```python
from build123d import *

# Parameters (mm, degrees)
F0_R     = 12.7
F1_DEPTH = 19.05
F2_R     = 2.54
F3_DEPTH = 12.7
F4_R     = 2.54
F4_R_2   = 2.674386
F5_DEPTH = 12.7


with BuildPart() as f1:
    # F0 (on Right) → F1 (new body)
    with BuildSketch(Plane.YZ):
        Circle(F0_R)
    extrude(amount=F1_DEPTH)

    # F2 (on face) → F3 (join)
    with BuildSketch(Plane.YZ.offset(19.05)):
        Circle(F2_R)
    extrude(amount=F3_DEPTH)

    # F4 (on face) → F5 (join)
    with BuildSketch(Plane(origin=(0, 0, 0), x_dir=(0, -1, 0), z_dir=(-1, 0, 0))):
        with Locations((-5.08, 0)):
            Circle(F4_R)
        with Locations((5.08, 0)):
            Circle(F4_R_2)
    extrude(amount=F5_DEPTH)


solid = f1.part
```
Verification items for the finished model (mm, model axes). A direction names the side the tool comes from. Give positions to 0.01 mm unless a question says otherwise; leave off trailing zeros. Order: outer loops, then holes, each group sorted by start corner. A loop starts at its lowest first (then second) coordinate and runs counter-clockwise, first axis right, second up. Notation, with made-up numbers: M 46,-38.75 L 89,-38.75 A22 ccw 89,-30.75 Z; hole C -33,71 d3. An arc over 180 degrees is marked long. Return JSON: item names as keys, results as strings. Group by question number.
1) Section check B-B on x = 15. Record the cut outline in (y, z).
2) Mould release check, pull along Y, two halves, no side actions. Record for faces 1 (the face through (9.39, -2.75, -12.4)), 2 (the face through (-12.7, 5, 0)), 3 (the face through (-6.261, 7.096, -1.546)): pulls with the +Y half, pulls with the -Y half, needs draft (parallel to the pull), parting line crosses it, or undercut.
3) Section check D-D on y = -5.08. Record the cut outline in (x, z), and give its area (3 significant figures).
4) Go/stop test with flat-tipped pins: pin 1 Ø10 at (y, z) = (-10, -6.5) entering from +X; pin 2 Ø4 at (y, z) = (-4, 6) entering from -X; pin 3 Ø2 at (x, z) = (-3, -3) entering from -Y. Record where each tip stops, or that it passes through.
5) Scan lines: line 1 (X direction, y = -7.25, z = 0.5); line 2 (X direction, y = -1.5, z = -4.75); line 3 (Y direction, x = 18, z = -11.5). Record each from-to range of solid material in increasing order.
6) Access from +Z, -Z, +X, -X, +Y, -Y to the whole of each face (thin tool, end or side, straight path). Record for faces 4 (the face through (31.75, 0, 0)), 5 (the face through (25.31, -0.33, 2.52)), 6 (the face through (-6.26, -2.41, 0.12)).
7) Section check A-A on y = 0. Record the cut outline in (x, z), and give its area (3 significant figures).
8) Section check C-C on z = -5.75. Record the cut outline in (x, y).
Answer block:
{
 "1": {"outline": "C 0,0 d25.4"},
 "2": {"face 1": "parting line crosses it", "face 2": "needs draft", "face 3": "undercut"},
 "3": {"outline": "M -12.7,-2.67 L 0,-2.67 L 0,-11.64 L 19.05,-11.64 L 19.05,11.64 L 0,11.64 L 0,2.67 L -12.7,2.67 Z", "area": "511 mm^2"},
 "4": {"pin 1": "stops at x = 19.05", "pin 2": "stops at x = 0", "pin 3": "stops at y = -6.86"},
 "5": {"line 1": "x = -12.7 to 19.05", "line 2": "x = 0 to 19.05", "line 3": "y = -5.39 to 5.39"},
 "6": {"face 4": "+Z, -Z, +X, +Y, -Y", "face 5": "+X", "face 6": "-X"},
 "7": {"outline": "M 0,-12.7 L 19.05,-12.7 L 19.05,-2.54 L 31.75,-2.54 L 31.75,2.54 L 19.05,2.54 L 19.05,12.7 L 0,12.7 Z", "area": "548 mm^2"},
 "8": {"outline": "M 0,-11.32 L 19.05,-11.32 L 19.05,11.32 L 0,11.32 Z"}
}
